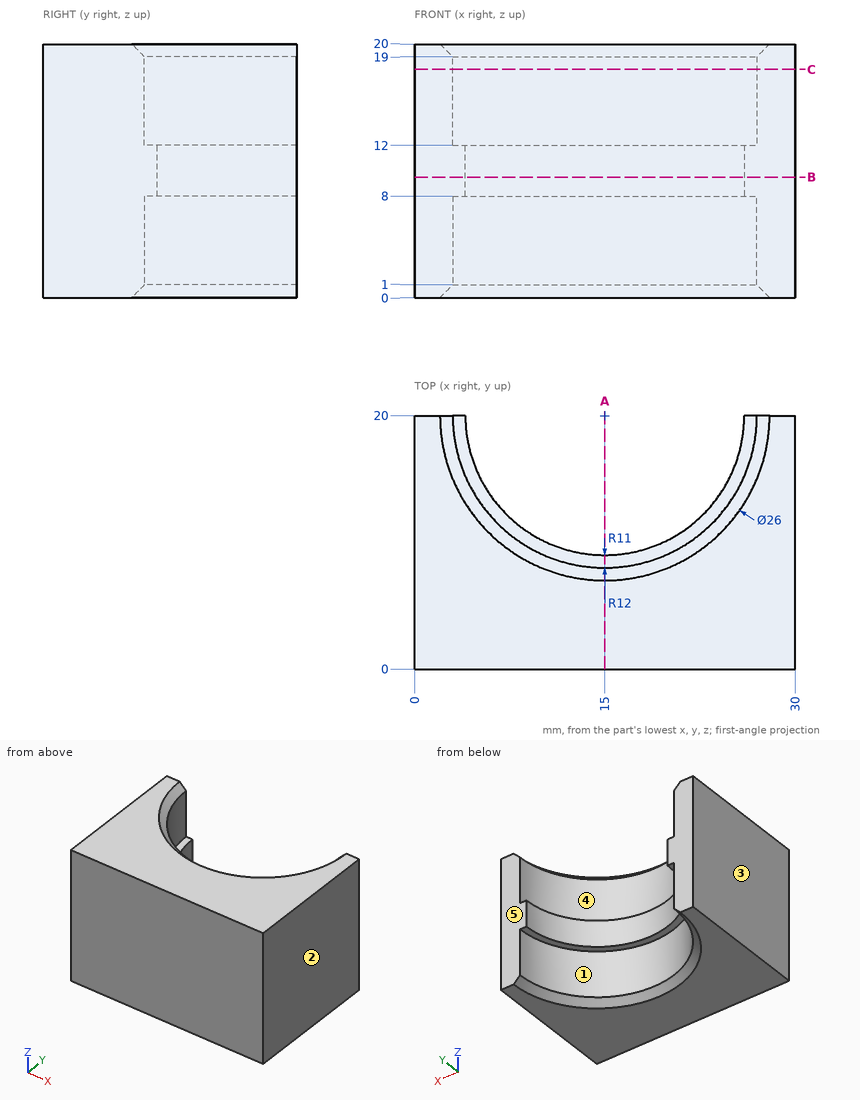
Geometry: see drawing. Coordinates: mm, zero at the bounding-box minimum. A direction names the side the tool comes from. Coordinates: 2 decimals unless noted, no trailing zeros. Write each loop counter-clockwise with the first axis right and the second up, starting at its lowest first coordinate (ties: lowest second). Pieces come first, ordered by that corner, then holes.
1) Section A-A on x = 15. Output: boundary loops of the cut face in (y, z).
2) Section B-B on z = 9.5. Output: boundary loops of the cut face in (x, y), and give its area (3 significant figures).
3) Material intervals for line 1 along X through (y, z) = (15.25, 6.5); line 2 along X through (y, z) = (19, 7.75); line 3 along Y through (x, z) = (11, 17), sorted ascending.
4) Pin query (flat end, axial travel): pin 1 Ø9.5 at (x, y) = (19.5, 15) entering from -Z; pin 2 Ø6 at (x, y) = (10.5, 15) entering from +Z. Return the tip coordinate at first contact, or that it passes through.
5) Set-up query: the marked faces 4 and 5. Return all of +Z, -Z, +X, -X, +Y, -Y with unobstructed straight access to the full face (end or side cutting, diameter ignored); none if empty.
6) Mould query, pull axis X, two halves, no side actions, for the marked faces 1, 2 and 3. Classes: pulls with the +X half, pulls with the -X half, needs draft (parallel to the pull), parting line crosses it, or undercut.
7) Section C-C on z = 18. Output: boundary loops of the cut face in (x, y).
Check result:
1. outline: (0, 0) - (7, 0) - (8, 1) - (8, 8) - (9, 8) - (9, 12) - (8, 12) - (8, 19) - (7, 20) - (0, 20) - close
2. outline: (0, 0) - (30, 0) - (30, 20) - (26, 20) arc R11 cw to (4, 20) - (0, 20) - close
2. area: 410 mm2
3. line 1: x = 0 to 3.98, 26.02 to 30
3. line 2: x = 0 to 3.04, 26.96 to 30
3. line 3: y = 0 to 8.69
4. pin 1: stops at z = 8
4. pin 2: passes through
5. face 4: +Z, +Y
5. face 5: +Z, -Z, +X, -X, +Y
6. face 1: undercut
6. face 2: pulls with the +X half
6. face 3: pulls with the -X half
7. outline: (0, 0) - (30, 0) - (30, 20) - (27, 20) arc R12 cw to (3, 20) - (0, 20) - close
